Build history of the part. All positions in model axes, mm. Give positions to 0.01 mm unless a question says otherwise; leave off trailing zeros. Order: outer loops, then holes, each group sorted by start corner. A loop starts at its lowest first (then second) coordinate and runs counter-clockwise, first axis right, second up. Notation, with made-up numbers: M -4,49 L 26,49 A23 ccw 26,87 Z; hole C -7.75,-0.75 d9. An arc over 180 degrees is marked long. Use CSV: the item, a comma, the result in double quotes. Start each with the question number.
Item 1: Band-saw the part on C-C on x = 84. Write the cut outline in (y, z), plus the area to 3 significant figures.
Item 2: Band-saw the part on B-B on y = -5. Write the cut outline in (x, z), plus the area to 3 significant figures.
Item 3: Pin check, flat tips, straight feed: P1, Ø2, axis at x = 23.5, y = -38, coming from the -Z side; P2, Ø3, axis at x = 67.5, y = 10, coming from the +Z side. Stop position of each tip, or through.
Item 4: Band-saw the part on A-A on x = 24.2. Give the number of separate pieces and of enclosed holes in the cut face, plus the area to 3 significant figures.
Item 5: Wall check: line 1 along Y through (x, z) = (-24, 2.35); line 2 along Y through (x, z) = (24.2, 2.2); line 3 along Z through (x, y) = (83.5, 43). Give the ranges that are in metal, low to high.
from build123d import *

# Parameters (mm, degrees)
F0_W     = 148
F0_H     = 122
F0_W_2   = 64
F0_H_2   = 102
F0_W_3   = 54
F0_H_3   = 82
F0_R     = 5
F0_R_2   = 3.5
F0_R_3   = 1.6
F1_DEPTH = 5
F2_DEPTH = 9
F3_DEPTH = 3
F4_R     = 3


with BuildPart() as f1:
    # F0 (on Top) → F1 (new body)
    with BuildSketch(Plane.XY):
        with Locations((32, 0)):
            Rectangle(F0_W, F0_H)
        Rectangle(F0_W_2, F0_H_2, mode=Mode.SUBTRACT)
        with Locations((69, 0)):
            Rectangle(F0_W_3, F0_H_3, mode=Mode.SUBTRACT)
        Rectangle(F0_W_2, F0_H_2)
        with Locations((-24.15, -35.65)):
            Circle(F0_R, mode=Mode.SUBTRACT)
        with Locations((24.2, -36.9)):
            Circle(F0_R, mode=Mode.SUBTRACT)
        with Locations((-24, 39.05)):
            Circle(F0_R, mode=Mode.SUBTRACT)
        with Locations((24.2, 45.25)):
            Circle(F0_R, mode=Mode.SUBTRACT)
        with Locations((69, 0)):
            Rectangle(F0_W_3, F0_H_3)
        with Locations((24.2, -36.9)):
            Circle(F0_R)
        with Locations((24.2, -36.9)):
            Circle(F0_R_2, mode=Mode.SUBTRACT)
        with Locations((-24.15, -35.65)):
            Circle(F0_R)
        with Locations((-24.15, -35.65)):
            Circle(F0_R_2, mode=Mode.SUBTRACT)
        with Locations((-24, 39.05)):
            Circle(F0_R)
        with Locations((-24, 39.05)):
            Circle(F0_R_2, mode=Mode.SUBTRACT)
        with Locations((24.2, 45.25)):
            Circle(F0_R)
        with Locations((24.2, 45.25)):
            Circle(F0_R_2, mode=Mode.SUBTRACT)
        with Locations((-24.15, -35.65)):
            Circle(F0_R_2)
        with Locations((-24.15, -35.65)):
            Circle(F0_R_3, mode=Mode.SUBTRACT)
        with Locations((24.2, -36.9)):
            Circle(F0_R_2)
        with Locations((24.2, -36.9)):
            Circle(F0_R_3, mode=Mode.SUBTRACT)
        with Locations((24.2, 45.25)):
            Circle(F0_R_2)
        with Locations((24.2, 45.25)):
            Circle(F0_R_3, mode=Mode.SUBTRACT)
        with Locations((-24, 39.05)):
            Circle(F0_R_2)
        with Locations((-24, 39.05)):
            Circle(F0_R_3, mode=Mode.SUBTRACT)
    extrude(amount=F1_DEPTH)

    # F0 (on Top) → F2 (join)
    with BuildSketch(Plane.XY):
        with Locations((24.2, -36.9)):
            Circle(F0_R)
        with Locations((24.2, -36.9)):
            Circle(F0_R_2, mode=Mode.SUBTRACT)
        with Locations((-24.15, -35.65)):
            Circle(F0_R)
        with Locations((-24.15, -35.65)):
            Circle(F0_R_2, mode=Mode.SUBTRACT)
        with Locations((-24, 39.05)):
            Circle(F0_R)
        with Locations((-24, 39.05)):
            Circle(F0_R_2, mode=Mode.SUBTRACT)
        with Locations((24.2, 45.25)):
            Circle(F0_R)
        with Locations((24.2, 45.25)):
            Circle(F0_R_2, mode=Mode.SUBTRACT)
        with Locations((-24, 39.05)):
            Circle(F0_R_2)
        with Locations((-24, 39.05)):
            Circle(F0_R_3, mode=Mode.SUBTRACT)
        with Locations((24.2, 45.25)):
            Circle(F0_R_2)
        with Locations((24.2, 45.25)):
            Circle(F0_R_3, mode=Mode.SUBTRACT)
        with Locations((24.2, -36.9)):
            Circle(F0_R_2)
        with Locations((24.2, -36.9)):
            Circle(F0_R_3, mode=Mode.SUBTRACT)
        with Locations((-24.15, -35.65)):
            Circle(F0_R_2)
        with Locations((-24.15, -35.65)):
            Circle(F0_R_3, mode=Mode.SUBTRACT)
    extrude(amount=F2_DEPTH)

    # F0 (on Top) → F3 (cut)
    with BuildSketch(Plane.XY):
        with Locations((24.2, -36.9)):
            Circle(F0_R_2)
        with Locations((24.2, -36.9)):
            Circle(F0_R_3, mode=Mode.SUBTRACT)
        with Locations((-24.15, -35.65)):
            Circle(F0_R_2)
        with Locations((-24.15, -35.65)):
            Circle(F0_R_3, mode=Mode.SUBTRACT)
        with Locations((-24, 39.05)):
            Circle(F0_R_2)
        with Locations((-24, 39.05)):
            Circle(F0_R_3, mode=Mode.SUBTRACT)
        with Locations((24.2, 45.25)):
            Circle(F0_R_2)
        with Locations((24.2, 45.25)):
            Circle(F0_R_3, mode=Mode.SUBTRACT)
    extrude(amount=F3_DEPTH, mode=Mode.SUBTRACT)

    # F4
    f4_edges = [f1.edges().sort_by_distance(p)[0] for p in [
        (19.2, -36.9, 5),
        (19.2, 45.25, 5),
        (-29.15, -35.65, 5),
        (-29, 39.05, 5),
    ]]
    fillet(f4_edges, radius=F4_R)


solid = f1.part
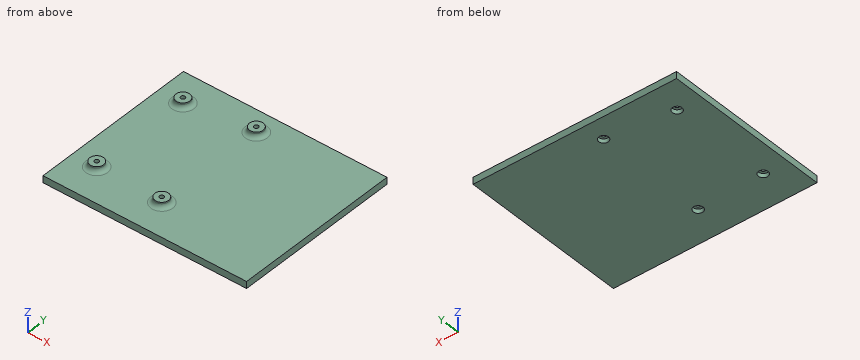
Model answer:
1,outline,"M -61,0 L 61,0 L 61,5 L -61,5 Z"
1,area,"610 mm^2"
2,outline,"M -42,0 L 106,0 L 106,5 L -42,5 Z"
2,area,"740 mm^2"
3,P1,"stops at z = 3"
3,P2,"stops at z = 5"
4,separate pieces,"3"
4,enclosed holes,"0"
4,area,"617 mm^2"
5,line 1,"y = -61 to -39.15, -32.15 to 35.55, 42.55 to 61"
5,line 2,"y = -61 to -40.4, -33.4 to 41.75, 48.75 to 61"
5,line 3,"z = 0 to 5"
